```python
from build123d import *

# Parameters (mm, degrees)
SKETCH1_R           = 11.5
SKETCH1_R_2         = 2
BOSS_EXTRUDE1_DEPTH = 3
SKETCH2_W           = 50
SKETCH2_H           = 54
BOSS_EXTRUDE2_DEPTH = 3
FILLET1_R           = 4
FILLET2_R           = 2
BOSS_EXTRUDE3_DEPTH = 3


with BuildPart() as part:
    # Sketch1 → Boss-Extrude1 (new body)
    with BuildSketch(Plane(origin=(0, 0, 0), x_dir=(1, 0, 0), z_dir=(0, 1, 0))):
        Polygon((21, 23.797619048), (25, 19.797619048), (25, -24.202380952), (-25, -24.202380952), (-25, 19.797619048), (-21, 23.797619048), align=None)
        with Locations(Location((0, 2.797619048, 0), (0, 0, 270))):
            Circle(SKETCH1_R, mode=Mode.SUBTRACT)
        with Locations(Location((-15, 19, 0), (0, 0, 270))):
            Circle(SKETCH1_R_2, mode=Mode.SUBTRACT)
        with Locations(Location((15, 18.797619048, 0), (0, 0, 270))):
            Circle(SKETCH1_R_2, mode=Mode.SUBTRACT)
        with Locations(Location((15, -12.202380952, 0), (0, 0, 270))):
            Circle(SKETCH1_R_2, mode=Mode.SUBTRACT)
        with Locations(Location((-15, -12.202380952, 0), (0, 0, 270))):
            Circle(SKETCH1_R_2, mode=Mode.SUBTRACT)
    extrude(amount=BOSS_EXTRUDE1_DEPTH)

    # Sketch2 → Boss-Extrude2 (add)
    with BuildSketch(Plane.XY.offset(24.202380952)):
        with Locations((0, 27)):
            Rectangle(SKETCH2_W, SKETCH2_H)
        with BuildLine():
            Line((-17.5, 43), (-17.5, 12))
            ThreePointArc((-17.5, 12), (-15.5, 10), (-13.5, 12))
            Line((-13.5, 12), (-13.5, 43))
            ThreePointArc((-13.5, 43), (-15.5, 45), (-17.5, 43))
        make_face(mode=Mode.SUBTRACT)
        with BuildLine():
            Line((12.5, 43), (12.5, 12))
            ThreePointArc((12.5, 12), (14.5, 10), (16.5, 12))
            Line((16.5, 12), (16.5, 43))
            ThreePointArc((16.5, 43), (14.5, 45), (12.5, 43))
        make_face(mode=Mode.SUBTRACT)
    extrude(amount=BOSS_EXTRUDE2_DEPTH)

    # Fillet1
    fillet1_edges = [part.edges().sort_by_distance(p)[0] for p in [
        (0, 0, 27.202380952),
    ]]
    fillet(fillet1_edges, radius=FILLET1_R)

    # Fillet2
    fillet2_edges = [part.edges().sort_by_distance(p)[0] for p in [
        (0, 3, 24.202380952),
    ]]
    fillet(fillet2_edges, radius=FILLET2_R)

    # Sketch6 → Boss-Extrude3 (add)
    with BuildSketch(Plane(origin=(25, 0, 0), x_dir=(0, 0, -1), z_dir=(1, 0, 0))):
        Polygon((-24.202380952, 3), (-24.202380952, 17), (-4.202380952, 3), align=None)
    boss_extrude3 = extrude(amount=-BOSS_EXTRUDE3_DEPTH)

    # Mirror1: Boss-Extrude3 across plane
    add(boss_extrude3.mirror(Plane(origin=(0, 0, 0), x_dir=(0, 0, 1), z_dir=(1, 0, 0))))


solid = part.part
```
The listing builds one solid part. Answer for the finished solid, in the listing's coordinates (mm). A direction names the side the tool comes from. Round coordinates to 2 decimals unless told otherwise and drop trailing zeros. Write each loop counter-clockwise with the first axis right and the second up, starting at its lowest first coordinate (ties: lowest second). Pieces come first, ordered by that corner, then holes. Notation, with made-up numbers: (31, 49) -> (63, 49) arc R9 cw to (63, 66) -> close; hole circle Ø7 at (65, 50). An arc over 180 degrees is marked (long way). Answer as a JSON object with one key per item and string values. Group by question number.
Q1. Each of these flat-tipped pins is pushed along its axis until it touches: pin 1 Ø24.5 at (x, y) = (2, 33) entering from -Z; pin 2 Ø3 at (x, z) = (-20, -6.5) entering from +Y; pin 3 Ø4 at (y, z) = (16, 16) entering from -X; pin 4 Ø6 at (x, z) = (11.5, 20) entering from +Y. Where does it stop, or does it pass through?
Q2. Section B-B (x = 0) is taken. Write down the section's boundary in (y, z), plus the area to 3 significant figures.
Q3. Determine the mould class of faces 4 (the face through (0, 0, 10)), 5 (the face through (-23.521, 10.098, 14.342)), 6 (the face through (0, 30, 24.202)), 7 (the face through (-17.5, 28, 26)) for opening direction Y: pulls with the +Y half, pulls with the -Y half, needs draft (parallel to the pull), parting line crosses it, or undercut.
Q4. Which of the six approach directions +Z, -Z, +X, -X, +Y, -Y give full straight-line access (tool end or side, diameter ignored) to faces 1 (the face through (-13, 1, -19)), 2 (the face through (-15.5, 10, 25.7)), 3 (the face through (0, 3, 9))?
Q5. Straight lines are drawn through the part: line 1 along X through (y, z) = (11.5, 23.5); line 2 along Y through (x, z) = (-20, -17.5); line 3 along Z through (x, y) = (19, 30.5). For each, find the intervals that lie inside material, in ascending order.
Q6. Section A-A (y = 32.5) is taken. Write down the section's boundary in (x, z), plus the area to 3 significant figures.
Q7. Section C-C (z = -7) is taken. Write down the section's boundary in (x, y), plus the area to 3 significant figures.
Q8. Section D-D (x = 15) is taken. Write down the section's boundary in (y, z).
Check values:
{
 "1": {"pin 1": "z = 24.2", "pin 2": "y = 3", "pin 3": "through", "pin 4": "y = 3.17"},
 "2": {"outline": "(0, -23.8) -> (3, -23.8) -> (3, -14.3) -> (0, -14.3) -> close; (0, 8.7) -> (3, 8.7) -> (3, 22.2) arc R2 cw to (5, 24.2) -> (54, 24.2) -> (54, 27.2) -> (4, 27.2) arc R4 ccw to (0, 23.2) -> close", "area": "234 mm^2"},
 "3": {"face 4": "pulls with the -Y half", "face 5": "pulls with the +Y half", "face 6": "needs draft", "face 7": "undercut"},
 "4": {"face 1": "+Y, -Y", "face 2": "+Z, -Z", "face 3": "-Z, +Y"},
 "5": {"line 1": "-25 to -22, 22 to 25", "line 2": "0 to 3", "line 3": "24.2 to 27.2"},
 "6": {"outline": "(-25, 24.2) -> (-17.5, 24.2) -> (-17.5, 27.2) -> (-25, 27.2) -> close; (-13.5, 24.2) -> (12.5, 24.2) -> (12.5, 27.2) -> (-13.5, 27.2) -> close; (16.5, 24.2) -> (25, 24.2) -> (25, 27.2) -> (16.5, 27.2) -> close", "area": "126 mm^2"},
 "7": {"outline": "(-25, 0) -> (-10.7, 0) -> (-10.7, 3) -> (-25, 3) -> close; (10.7, 0) -> (25, 0) -> (25, 3) -> (10.7, 3) -> close", "area": "85.8 mm^2"},
 "8": {"outline": "(0, -23.8) -> (3, -23.8) -> (3, -20.8) -> (0, -20.8) -> close; (0, -16.8) -> (3, -16.8) -> (3, 10.2) -> (0, 10.2) -> close; (0, 14.2) -> (3, 14.2) -> (3, 22.2) arc R2 cw to (5, 24.2) -> (10.06, 24.2) -> (10.06, 27.2) -> (4, 27.2) arc R4 ccw to (0, 23.2) -> close; (44.94, 24.2) -> (54, 24.2) -> (54, 27.2) -> (44.94, 27.2) -> close"}
}
